from build123d import *

# Parameters (mm, degrees)
SKETCH1_R           = 0.95
BOSS_EXTRUDE1_DEPTH = 18
SKETCH2_W           = 32
SKETCH2_H           = 82.41
CUT_EXTRUDE1_DEPTH  = 18
SKETCH3_R           = 3.75
BOSS_EXTRUDE2_DEPTH = 34


with BuildPart() as part:
    # Sketch1 → Boss-Extrude1 (new, symmetric)
    with BuildSketch(Plane(origin=(0, 0, 0), x_dir=(0, 0, -1), z_dir=(1, 0, 0))):
        with BuildLine():
            Line((0, 3.13), (31.1, 3.13))
            Line((31.1, 3.13), (46.4, 1.791423448))
            Line((46.4, 1.791423448), (63, -0.645051075))
            Line((63, -0.645051075), (70.82606591, -5.894041546))
            ThreePointArc((70.82606591, -5.894041546), (73.097461385, -6.814738199), (75.547517331, -6.750351941))
            Line((75.547517331, -6.750351941), (76.475855369, -6.531065029))
            ThreePointArc((76.475855369, -6.531065029), (79.176402306, -8.070534767), (77.831396153, -10.873012114))
            Line((77.831396153, -10.873012114), (70.486743317, -13.749263303))
            ThreePointArc((70.486743317, -13.749263303), (67.920640594, -14.150456708), (65.425410054, -13.429579543))
            Line((65.425410054, -13.429579543), (61.610342493, -11.348317948))
            ThreePointArc((61.610342493, -11.348317948), (60.047195579, -10.760330177), (58.382530932, -10.625981737))
            Line((58.382530932, -10.625981737), (37.275936798, -11.874727235))
            ThreePointArc((37.275936798, -11.874727235), (36.082237819, -11.362512436), (35.77777119, -10.099745108))
            Line((35.77777119, -10.099745108), (36.587860094, -6.605922434))
            ThreePointArc((36.587860094, -6.605922434), (36.310540144, -5.376298946), (35.17533219, -4.828409195))
            Line((35.17533219, -4.828409195), (7, -4.828409195))
            Line((7, -4.828409195), (-0.7040968, -3.049778303))
            ThreePointArc((-0.7040968, -3.049778303), (-3.109879908, 0.354326059), (0, 3.13))
        make_face()
        Circle(SKETCH1_R, mode=Mode.SUBTRACT)
        with Locations((77, -8.75)):
            Circle(SKETCH1_R, mode=Mode.SUBTRACT)
        with Locations((39.75, -8.75)):
            Circle(SKETCH1_R, mode=Mode.SUBTRACT)
        with Locations((44.1, -5.6)):
            Circle(SKETCH1_R, mode=Mode.SUBTRACT)
    extrude(amount=BOSS_EXTRUDE1_DEPTH, both=True)

    # Sketch2 → Cut-Extrude1 (cut, symmetric)
    with BuildSketch(Plane(origin=(0, 0, 0), x_dir=(1, 0, 0), z_dir=(0, 1, 0))):
        with Locations((0, 38.075)):
            Rectangle(SKETCH2_W, SKETCH2_H)
    extrude(amount=CUT_EXTRUDE1_DEPTH, both=True, mode=Mode.SUBTRACT)


with BuildPart() as cut_extrude1_piece_1:
    # of the separate pieces the step leaves, piece 1, a body of its own (cut_extrude1_pieces)
    add(part.part.solids().sort_by_distance((16, -4.828409195, -35.17533219))[0])



with BuildPart() as cut_extrude1_piece_2:
    # of the separate pieces the step leaves, piece 2, a body of its own (cut_extrude1_pieces)
    add(part.part.solids().sort_by_distance((-18, -4.828409195, -35.17533219))[0])


with BuildPart() as cut_extrude1_piece_1_1:
    add(cut_extrude1_piece_1.part)

    add(cut_extrude1_piece_2.part)  # Boss-Extrude2 merges Cut-Extrude1 piece 2
    # Sketch3 → Boss-Extrude2 (add)
    with BuildSketch(Plane(origin=(18, 0, 0), x_dir=(0, 0, -1), z_dir=(1, 0, 0))):
        with Locations((58.65, -5.75)):
            Circle(SKETCH3_R)
    extrude(amount=-BOSS_EXTRUDE2_DEPTH)


solid = cut_extrude1_piece_1_1.part
Verification items for the finished model (mm, model axes). A direction names the side the tool comes from. Round coordinates to 2 decimals unless told otherwise and drop trailing zeros. Loops run counter-clockwise (first coordinate to the right, second up) from the corner with the lowest first, then second, coordinate; pieces in that order, holes last. Notation, with made-up numbers: (21, -12.75) - (30, -12.75) arc R9 ccw to (30, 1.25) - close; hole circle Ø3 at (-26, 17). An arc over 180 degrees is marked (long way). Use one line per item in the form item = value.
1. Section check D-D on z = -44.1. Record the cut outline in (x, y).
A:
outline = (-18, -11.47) - (-16, -11.47) - (-16, -6.55) - (-18, -6.55) - close; (-18, -4.65) - (-16, -4.65) - (-16, 1.99) - (-18, 1.99) - close; (16, -11.47) - (18, -11.47) - (18, -6.55) - (16, -6.55) - close; (16, -4.65) - (18, -4.65) - (18, 1.99) - (16, 1.99) - close
2. Section check C-C on x = -3. Record the cut outline in (y, z).
A:
outline = circle Ø7.5 at (-5.75, -58.65)
3. Gauge pin test, flat ends, axial feed: pin 1 Ø8 at (x, z) = (6.5, -53) entering from -Y; pin 2 Ø1.1 at (y, z) = (-8.75, -39.75) entering from -X; pin 3 Ø8 at (y, z) = (-7.5, -10) entering from +X; pin 4 Ø10 at (x, y) = (-6, -9) entering from +Z. Record the tip position at first contact, or that the pin passes through.
A:
pin_1 = -9.12
pin_2 = through
pin_3 = 18
pin_4 = -54.9
4. Section check B-B on y = -8.75. Record the cut outline in (x, z), and give its area (3 significant figures).
A:
outline = (-18, -79.28) - (-16, -79.28) - (-16, -77.95) - (-18, -77.95) - close; (-18, -76.05) - (-16, -76.05) - (-16, -60.9) - (16, -60.9) - (16, -76.05) - (18, -76.05) - (18, -40.7) - (16, -40.7) - (16, -56.4) - (-16, -56.4) - (-16, -40.7) - (-18, -40.7) - close; (-18, -38.8) - (-16, -38.8) - (-16, -36.09) - (-18, -36.09) - close; (16, -79.28) - (18, -79.28) - (18, -77.95) - (16, -77.95) - close; (16, -38.8) - (18, -38.8) - (18, -36.09) - (16, -36.09) - close
area = 302 mm²
5. Draft check along Y on faces 4 (the cylindrical face through (-17.01, 0.04, 0.95)), 5 (the flat face through (-18, -3, -39)), 6 (the flat face through (-17, 3.13, -15)). Enter one of: pulls with the +Y half, pulls with the -Y half, needs draft (parallel to the pull), parting line crosses it, or undercut.
A:
face_4 = undercut
face_5 = needs draft
face_6 = pulls with the +Y half
6. Access from +Z, -Z, +X, -X, +Y, -Y to the whole of each face (thin tool, end or side, straight path). Record for faces 1 (the cylindrical face through (17.014, -10.765, -60.07)), 2 (the cylindrical face through (0.224, -4.624, -62.227)), 3 (the flat face through (17, 3.13, -15)).
A:
face_1 = +X, -X, -Y
face_2 = none
face_3 = +Z, -Z, +X, -X, +Y
7. Scan lines: probe 1 along X at (y, z) = (-3.75, -31.5); probe 2 along Z at (x, y) = (17.25, -8.75); probe 3 along Y at (x, z) = (17.3, -77). Record each from-to range of solid material in increasing order.
A:
probe_1 = -18 to -16, 16 to 18
probe_2 = -79.28 to -77.95, -76.05 to -40.7, -38.8 to -36.09
probe_3 = -11.2 to -9.7, -7.8 to -6.47
8. Section check A-A on z = -29. Record the cut outline in (x, y).
A:
outline = (-18, -4.83) - (-16, -4.83) - (-16, 3.13) - (-18, 3.13) - close; (16, -4.83) - (18, -4.83) - (18, 3.13) - (16, 3.13) - close
